Input: part model. Units: mm. Frame: model coordinates. Face numbers are marked on the shaded views. A direction names the side the tool comes from. Coordinates: 2 decimals unless noted, no trailing zeros. Loops run counter-clockwise (first coordinate to the right, second up) from the corner with the lowest first, then second, coordinate; pieces in that order, holes last. Notation, with made-up numbers: (-0.75, 28) - (13.25, 28) arc R13 ccw to (13.25, 33) - close; hole circle Ø9 at (-35, 10). An arc over 180 degrees is marked (long way). Answer as CSV lines item,"result". Start each with the question number.
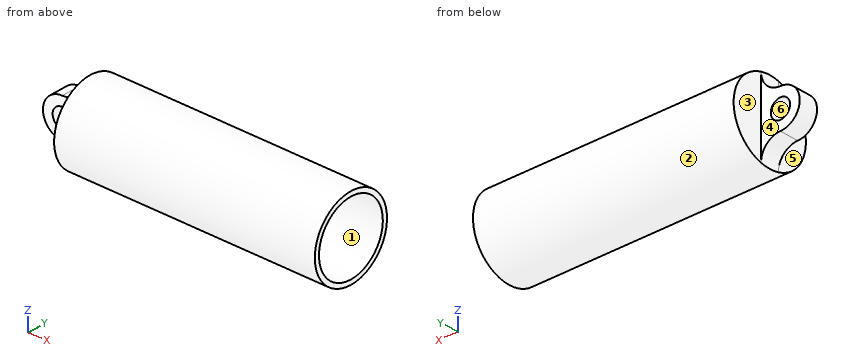
```python
from build123d import *

# Parameters (mm, degrees)
CYLINDER071_R           = 6
CYLINDER071_DEPTH       = 10
CYLINDER071_ROLL_ANGLE  = 90
CYLINDER072_R           = 6
CYLINDER072_DEPTH       = 10
CYLINDER072_ROLL_ANGLE  = 90
BOX003_W                = 6
BOX003_H                = 10
BOX003_DEPTH            = 38
BOX002_W                = 14
BOX002_H                = 10
BOX002_DEPTH            = 38
CYLINDER070_R           = 6
CYLINDER070_DEPTH       = 10
CYLINDER070_ROLL_ANGLE  = 90
CYLINDER006_R           = 11.05
CYLINDER006_DEPTH       = 75.8
CYLINDER006_PITCH_ANGLE = 90
CYLINDER018_R           = 3
CYLINDER018_DEPTH       = 30
CYLINDER018_ROLL_ANGLE  = 90
BOX001_W                = 14
BOX001_H                = 15
BOX001_DEPTH            = 30
BOX_W                   = 14
BOX_H                   = 15
BOX_DEPTH               = 30
CYLINDER005_R           = 12.5
CYLINDER005_DEPTH       = 95
CYLINDER005_PITCH_ANGLE = 90


with BuildPart() as cylinder076:
    # Cylinder071 → Cylinder071 (new body)
    with BuildSketch(Plane.XY):
        Circle(CYLINDER071_R)
    extrude(amount=CYLINDER071_DEPTH)


with BuildPart() as cylinder076_1:
    # Cylinder071 roll: moved
    add(cylinder076.part.rotate(Axis((0, 0, 0), (1, 0, 0)), CYLINDER071_ROLL_ANGLE))


with BuildPart() as cylinder076_2:
    # Cylinder071 placement: moved
    add(cylinder076_1.part.moved(Location((-9, 5, -12))))


with BuildPart() as cylinder077:
    # Cylinder072 → Cylinder072 (new body)
    with BuildSketch(Plane.XY):
        Circle(CYLINDER072_R)
    extrude(amount=CYLINDER072_DEPTH)


with BuildPart() as cylinder077_1:
    # Cylinder072 roll: moved
    add(cylinder077.part.rotate(Axis((0, 0, 0), (1, 0, 0)), CYLINDER072_ROLL_ANGLE))


with BuildPart() as cylinder077_2:
    # Cylinder072 placement: moved
    add(cylinder077_1.part.moved(Location((-9, 5, 0))))


with BuildPart() as cube003:
    # Box003 → Box003 (new body)
    with BuildSketch(Plane(origin=(-9, -5, -19), x_dir=(1, 0, 0), z_dir=(0, 0, 1))):
        with Locations((3, 5)):
            Rectangle(BOX003_W, BOX003_H)
    extrude(amount=BOX003_DEPTH)


with BuildPart() as cut065:
    # Box002 → Box002 (new body)
    with BuildSketch(Plane(origin=(-17, -5, -19), x_dir=(1, 0, 0), z_dir=(0, 0, 1))):
        with Locations((7, 5)):
            Rectangle(BOX002_W, BOX002_H)
    extrude(amount=BOX002_DEPTH)

    # Cut064: cut Cube003
    add(cube003.part, mode=Mode.SUBTRACT)

    # Cut065: cut Cylinder077
    add(cylinder077_2.part, mode=Mode.SUBTRACT)


with BuildPart() as fusion015:
    # Cylinder070 → Cylinder070 (new body)
    with BuildSketch(Plane.XY):
        Circle(CYLINDER070_R)
    extrude(amount=CYLINDER070_DEPTH)


with BuildPart() as fusion015_1:
    # Cylinder070 roll: moved
    add(fusion015.part.rotate(Axis((0, 0, 0), (1, 0, 0)), CYLINDER070_ROLL_ANGLE))


with BuildPart() as fusion015_2:
    # Cylinder070 placement: moved
    add(fusion015_1.part.moved(Location((-9, 5, 12))))

    # Fusion015: union Cylinder076, Cut065
    add(cylinder076_2.part)
    add(cut065.part)


with BuildPart() as cylinder004:
    # Cylinder006 → Cylinder006 (new body)
    with BuildSketch(Plane.XY):
        Circle(CYLINDER006_R)
    extrude(amount=CYLINDER006_DEPTH)


with BuildPart() as cylinder004_1:
    # Cylinder006 pitch: moved
    add(cylinder004.part.rotate(Axis((0, 0, 0), (0, 1, 0)), CYLINDER006_PITCH_ANGLE))


with BuildPart() as cylinder004_2:
    # Cylinder006 placement: moved
    add(cylinder004_1.part.moved(Location((2.2, 0, 0))))


with BuildPart() as cylinder016:
    # Cylinder018 → Cylinder018 (new body)
    with BuildSketch(Plane.XY):
        Circle(CYLINDER018_R)
    extrude(amount=CYLINDER018_DEPTH)


with BuildPart() as cylinder016_1:
    # Cylinder018 roll: moved
    add(cylinder016.part.rotate(Axis((0, 0, 0), (1, 0, 0)), CYLINDER018_ROLL_ANGLE))


with BuildPart() as cylinder016_2:
    # Cylinder018 placement: moved
    add(cylinder016_1.part.moved(Location((-9, 15, 0))))


with BuildPart() as cube001:
    # Box001 → Box001 (new body)
    with BuildSketch(Plane(origin=(-17, -18, -15), x_dir=(1, 0, 0), z_dir=(0, 0, 1))):
        with Locations((7, 7.5)):
            Rectangle(BOX001_W, BOX001_H)
    extrude(amount=BOX001_DEPTH)


with BuildPart() as cube:
    # Box → Box (new body)
    with BuildSketch(Plane(origin=(-17, 3, -15), x_dir=(1, 0, 0), z_dir=(0, 0, 1))):
        with Locations((7, 7.5)):
            Rectangle(BOX_W, BOX_H)
    extrude(amount=BOX_DEPTH)


with BuildPart() as batterycap2:
    # Cylinder005 → Cylinder005 (new body)
    with BuildSketch(Plane.XY):
        Circle(CYLINDER005_R)
    extrude(amount=CYLINDER005_DEPTH)


with BuildPart() as batterycap2_1:
    # Cylinder005 pitch: moved
    add(batterycap2.part.rotate(Axis((0, 0, 0), (0, 1, 0)), CYLINDER005_PITCH_ANGLE))


with BuildPart() as batterycap2_2:
    # Cylinder005 placement: moved
    add(batterycap2_1.part.moved(Location((-17, 0, 0))))

    # Cut010: cut Cube
    add(cube.part, mode=Mode.SUBTRACT)

    # Cut011: cut Cube001
    add(cube001.part, mode=Mode.SUBTRACT)

    # Cut012: cut Cylinder016
    add(cylinder016_2.part, mode=Mode.SUBTRACT)

    # Cut013: cut Cylinder004
    add(cylinder004_2.part, mode=Mode.SUBTRACT)

    # Cut066: cut Fusion015
    add(fusion015_2.part, mode=Mode.SUBTRACT)


solid = batterycap2_2.part
```
Item 1: Section query A-A, the plane y = 0. Output: boundary loops of the cut face in (x, z), and give its area (3 significant figures).
Item 2: Draft query along X for the marked faces 4, 5 and 6. Return one class per face: pulls with the +X half, pulls with the -X half, needs draft (parallel to the pull), parting line crosses it, or undercut.
Item 3: Section query B-B, the plane z = 0. Output: boundary loops of the cut face in (x, y).
Item 4: Section query D-D, the plane y = 4.5. Output: boundary loops of the cut face in (x, z), and give its area (3 significant figures).
Item 5: Section query C-C, the plane x = -8. Output: boundary loops of the cut face in (y, z), and give its area (3 significant figures).
Item 6: Contact query for flat-ended pins moving along their axis: P1, Ø6, axis at x = -10.5, z = 0.5, coming from the +Y side; P2, Ø3, axis at y = 6.5, z = -1, coming from the -X side; P3, Ø2, axis at x = 55, z = -1.5, coming from the +Y side. Output: stop coordinate, or through.
Item 7: Set-up query: the marked faces 1, 2 and 3. Return all of +Z, -Z, +X, -X, +Y, -Y with unobstructed straight access to the full face (end or side cutting, diameter ignored); none if empty.
Item 8: Material intervals for probe 1 along Z at (x, y) = (-9, 1.75); probe 2 along Y at (x, z) = (26, 0); probe 3 along Z at (x, y) = (26.5, -0.5), sorted ascending.
Response values:
1,outline,"(-9, -6) arc R6 cw to (-3.02, -12.5) - (78, -12.5) - (78, -11.05) - (2.2, -11.05) - (2.2, 11.05) - (78, 11.05) - (78, 12.5) - (-3.02, 12.5) arc R6 cw to (-9, 6) arc R6 ccw to start; hole circle Ø6 at (-9, 0)"
1,area,"466 mm²"
2,face 4,"needs draft"
2,face 5,"pulls with the -X half"
2,face 6,"undercut"
3,outline,"(-15, -3) - (-12, -3) - (-12, 3) - (-15, 3) - close; (-6, -3) - (-3, -3) - (-3, -12.5) - (78, -12.5) - (78, -11.05) - (2.2, -11.05) - (2.2, 11.05) - (78, 11.05) - (78, 12.5) - (-3, 12.5) - (-3, 3) - (-6, 3) - close"
4,outline,"(-3, -11.66) - (78, -11.66) - (78, -10.09) - (2.2, -10.09) - (2.2, 10.09) - (78, 10.09) - (78, 11.66) - (-3, 11.66) - close"
4,area,"359 mm²"
5,outline,"(-3, -6.08) - (3, -6.08) - (3, -2.83) - (-3, -2.83) - close; (-3, 2.83) - (3, 2.83) - (3, 6.08) - (-3, 6.08) - close"
5,area,"39.1 mm²"
6,P1,"stops at y = 3"
6,P2,"stops at x = -3"
6,P3,"stops at y = 12.49"
7,face 1,"+X"
7,face 2,"+X, -X"
7,face 3,"+Z, -Z, -X, +Y"
8,probe 1,"z = -6 to -3, 3 to 6"
8,probe 2,"y = -12.5 to -11.05, 11.05 to 12.5"
8,probe 3,"z = -12.49 to -11.04, 11.04 to 12.49"
